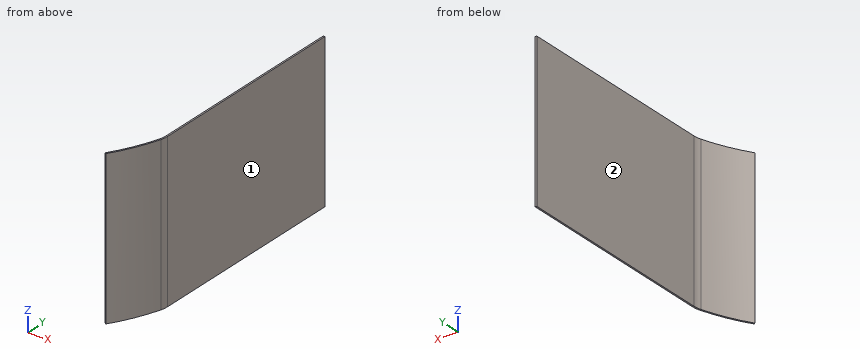
Autodesk Inventor part; units mm, degrees
ref_plane "YZ Plane" through (0, 0, 0) normal (1, 0, 0) x (0, 1, 0)
ref_plane "XZ Plane" through (0, 0, 0) normal (0, 1, 0) x (-1, 0, 0)
ref_plane "XY Plane" through (0, 0, 0) normal (0, 0, 1) x (1, 0, 0)
ref_plane "Work Plane1" through (0, 0, 0) normal (0, 0, 1) x (1, 0, 0)
sketch "Sketch1" plane through (0, 0, 0) normal (0, 0, 1) x (1, 0, 0)
  line L0 (-5.0952, -133.1293) -> (-4.7767, -132.9202) construction
  arc A0 (-5.0952, -133.1293) -> (-0.7466, -139.7544) centre (-1.0882, -135.2389) ccw construction
  line L1 (4.7811, 106.7831) -> (4.7811, -102.6288)
  arc A1 (-17.4789, -155.8337) -> (3.6681, -110.0654) centre (-174.5174, -55.5054) ccw
  line L2 (4.7811, 106.7831) -> (3.1936, 106.7831)
  line L3 (4.7811, -105.9343) -> (6.3686, -105.9343) construction
  line L4 (3.1936, -102.5821) -> (3.1936, 106.7831)
  line L5 (-17.4789, -155.8337) -> (-18.8167, -154.979)
  line L6 (-174.5174, -55.5054) -> (-175.8552, -54.6508)
  line L7 (-174.5174, -55.5054) -> (-172.9299, -55.5054) construction
  arc A2 (-18.8167, -154.979) -> (2.0412, -110.1462) centre (-175.8552, -54.6508) ccw
  line L8 (3.1936, -105.9343) -> (3.1936, -105.9468)
  arc A3 (2.0412, -110.1462) -> (3.1936, -102.5821) centre (-22.2064, -102.5821) ccw
  arc A4 (3.6681, -110.0654) -> (4.7811, -102.6288) centre (-20.6189, -102.6288) ccw
  point P0 (0, 0)
  point P1 (4.7811, -106.2883)
  dimension "d1" = 1.5875
  dimension "d6" = 1.5875
  dimension "d7" = 1.5875
  dimension "d8" = 147.426
  dimension "d13" = 25.4
extrude "Extrusion1" add sketch "Sketch1" against normal blind 158.75
properties part number "Intake main polycarb" material "Polycarbonate, Clear"
Geometry: final body of the model. Coordinates: model frame, mm. Face numbers are marked on the shaded views. A direction names the side the tool comes from. Round coordinates to 2 decimals unless told otherwise and drop trailing zeros. Order: outer loops, then holes, each group sorted by start corner. A loop starts at its lowest first (then second) coordinate and runs counter-clockwise, first axis right, second up. Notation, with made-up numbers: (-29.5, 2) -> (-11.5, 2) arc R25 ccw to (-11.5, 17) -> close; hole circle Ø9 at (-4, -35.5). An arc over 180 degrees is marked (long way). Put each result on its own line as item: value. Start each with the question number.
Q1. Section A-A on z = -77. Return the cut outline in (x, y).
Q2. First-contact query: pin 1 (10 mm diameter, centred on y = -59.5, z = -77.5, fed in from -X); pin 2 (12 mm diameter, centred on x = -7.5, z = -53.5, fed in from -Y); pin 3 (4 mm diameter, centred on x = -15.5, z = -138, fed in from +Y). Flat tips, straight axial feed; report the tip coordinate or a pass-through.
Q3. Section C-C on x = -4.75. Return the cut outline in (y, z).
Q4. Reachability of the marked faces 1 and 2 from +Z, -Z, +X, -X, +Y, -Y: full face, straight path, thin tool, end or side. Return the list, or none.
Q5. Section B-B on y = 78. Return the cut outline in (x, z).
Q6. Line query: probe 1 along X at (y, z) = (-71.5, -44); probe 2 along Y at (x, z) = (-16, -57); probe 3 along Y at (x, z) = (-6.5, -142.5). Output: solid intervals per line, ascending.
Ans:
1. outline: (-18.82, -154.98) -> (-17.48, -155.83) arc R186.35 ccw to (3.67, -110.07) arc R25.4 ccw to (4.78, -102.63) -> (4.78, 106.78) -> (3.19, 106.78) -> (3.19, -102.58) arc R25.4 cw to (2.04, -110.15) arc R186.36 cw to start
2. pin 1: stops at x = 3.19
2. pin 2: stops at y = -149.32
2. pin 3: stops at y = -146.13
3. outline: (-132.36, -158.75) -> (-128.47, -158.75) -> (-128.47, 0) -> (-132.36, 0) -> close
4. face 1: +Z, -Z, +X, +Y, -Y
4. face 2: +Z, -Z, -X, +Y
5. outline: (3.19, -158.75) -> (4.78, -158.75) -> (4.78, 0) -> (3.19, 0) -> close
6. probe 1: x = 3.19 to 4.78
6. probe 2: y = -153.48 to -150.43
6. probe 3: y = -136.11 to -132.4
